For this review, take the finished solid that the model builds, in its own axes (mm). A direction names the side the tool comes from. Coordinates: 2 decimals unless noted, no trailing zeros. Loops run counter-clockwise (first coordinate to the right, second up) from the corner with the lowest first, then second, coordinate; pieces in that order, holes last.
Autodesk Inventor part; units mm, degrees
ref_plane "YZ Plane" through (0, 0, 0) normal (1, 0, 0) x (0, 1, 0)
ref_plane "XZ Plane" through (0, 0, 0) normal (0, 1, 0) x (-1, 0, 0)
ref_plane "XY Plane" through (0, 0, 0) normal (0, 0, 1) x (1, 0, 0)
sketch "Sketch1" plane through (0, 0, 0) normal (0, 0, 1) x (1, 0, 0)
  line L0 (0, 12) -> (0, 0)
  line L1 (0, 0) -> (8.5, 0)
  line L2 (8.5, 0) -> (8.5, 6)
  line L3 (8.5, 6) -> (23.5, 6)
  line L4 (23.5, 6) -> (23.5, 0)
  line L5 (23.5, 0) -> (32, 0)
  line L6 (32, 0) -> (32, 12)
  line L7 (32, 12) -> (0, 12)
  dimension "d0" = 32
  dimension "d1" = 12
  dimension "d2" = 8.5
  dimension "d3" = 6
extrude "Extrusion1" add sketch "Sketch1" along normal blind 58.8
sketch "Sketch2" plane through (0, 12, 0) normal (0, 1, 0) x (1, 0, 0)
  line L0 (3.5, -41.9) -> (28.5, -41.9) construction
  line L1 (28.5, -41.9) -> (28.5, -16.9) construction
  line L2 (28.5, -16.9) -> (3.5, -16.9) construction
  line L3 (3.5, -16.9) -> (3.5, -41.9) construction
  circle A0 centre (3.5, -41.9) radius 1.5
  circle A1 centre (3.5, -16.9) radius 1.5
  circle A2 centre (28.5, -41.9) radius 1.5
  circle A3 centre (28.5, -16.9) radius 1.5
  line L4 (32, -58.8) -> (0, -58.8) construction
  line L5 (32, 0) -> (0, 0) construction
  line L6 (16, -41.9) -> (16, -58.8) construction
  line L7 (16, -16.9) -> (16, 0) construction
  dimension "d6" = 3
  dimension "d7" = 25
  dimension "d8" = 25
extrude "Extrusion2" cut sketch "Sketch2" against normal blind 4
sketch "Sketch3" plane through (0, 0, 58.8) normal (0, 0, 1) x (1, 0, 0)
  line L0 (8.5, 6) -> (23.5, 6)
  line L1 (32, 12) -> (0, 12)
  circle A0 centre (16, 9) radius 3
  point P0 (0, 0)
  point P1 (16, 12)
  dimension "d11" = 6
extrude "Extrusion3" add sketch "Sketch3" along normal blind 4.5
properties part number "MGN15H-Carrier"
Q1. Wall thickness on probe 1 along X at (y, z) = (11, 16.9); probe 2 along Z at (x, y) = (28.5, 10.6); probe 3 along X at (y, z) = (3.5, 29.5): over which ranges is each line inside the solid? List them lowest first.
Q2. Consider section A-A (y = 9). State the section outline as (x, z) points, then the cut area to 3 significant figures.
Q3. Consider section C-C (z = 16.9). State the section outline as (x, y) points.
Q4. Machinability: for faces 1 (the face through (3.305, 10.028, 40.413)), 2 (the face through (4, 0, 29)), 3 (the face through (13.79, 6.97, 61.02)), which of the approach directions +Z, -Z, +X, -X, +Y, -Y give a long, thin tool a straight path to every point of the face, cutting with its end or side? Answer none if there is none.
Q5. For pin 1 Ø1.5 at (x, z) = (29, 41.5) entering from +Y; pin 2 Ø1 at (x, z) = (12.5, 12.5) entering from -Y; pin 3 Ø1.5 at (x, y) = (10.5, 6) entering from +Z, all flat-tipped, find the tip position at first contact; note any pin that passes through.
Q6. Consider section D-D (y = 1.75). State the section outline as (x, z) points, then the cut area to 4 significant figures.
Q7. The part is to be moulded in two halves that separate along Z. For faces 4 (the face through (0, 6, 29)), 5 (the face through (16, 9, 63.3)), 6 (the face through (27, 10.03, 16.83)), say which applies: +Z half, -Z half, draft (parallel to the pull), parting line (faces both ways), or undercut.
Q8. Consider section B-B (x = 28.5). State the section outline as (y, z) points, then the cut area to 3 significant figures.
Model answer:
1. probe 1: x = 0 to 2, 5 to 27, 30 to 32
1. probe 2: z = 0 to 15.4, 18.4 to 40.4, 43.4 to 58.8
1. probe 3: x = 0 to 8.5, 23.5 to 32
2. outline: (0, 0) - (32, 0) - (32, 58.8) - (19, 58.8) - (19, 63.3) - (13, 63.3) - (13, 58.8) - (0, 58.8) - close; hole circle Ø3 at (3.5, 16.9); hole circle Ø3 at (3.5, 41.9); hole circle Ø3 at (28.5, 16.9); hole circle Ø3 at (28.5, 41.9)
2. area: 1,880 mm2
3. outline: (0, 0) - (8.5, 0) - (8.5, 6) - (23.5, 6) - (23.5, 0) - (32, 0) - (32, 12) - (30, 12) - (30, 8) - (27, 8) - (27, 12) - (5, 12) - (5, 8) - (2, 8) - (2, 12) - (0, 12) - close
4. face 1: +Y
4. face 2: +Z, -Z, +X, -X, -Y
4. face 3: +Z
5. pin 1: stops at y = 8
5. pin 2: stops at y = 6
5. pin 3: stops at z = 58.8
6. outline: (0, 0) - (8.5, 0) - (8.5, 58.8) - (0, 58.8) - close; (23.5, 0) - (32, 0) - (32, 58.8) - (23.5, 58.8) - close
6. area: 1,000 mm2
7. face 4: draft
7. face 5: +Z half
7. face 6: undercut
8. outline: (0, 0) - (12, 0) - (12, 15.4) - (8, 15.4) - (8, 18.4) - (12, 18.4) - (12, 40.4) - (8, 40.4) - (8, 43.4) - (12, 43.4) - (12, 58.8) - (0, 58.8) - close
8. area: 682 mm2
